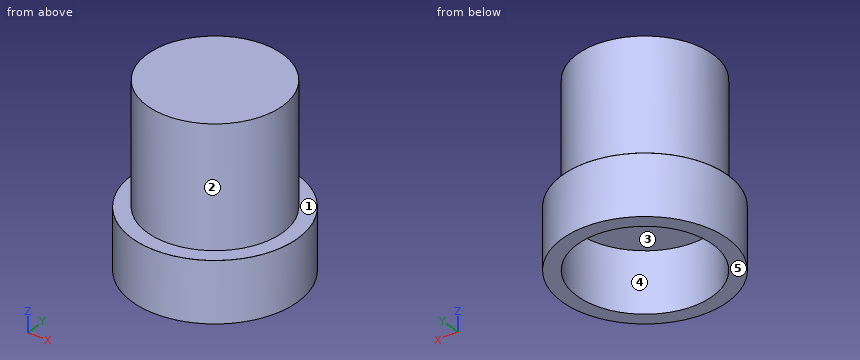
from build123d import *

# Parameters (mm, degrees)
F0_R          = 14.2875
F1_DEPTH      = 25.4
F0_R_2        = 17.4625
F2_DEPTH      = 12.7
F2_DEPTH_BACK = 0.0254


with BuildPart() as f1:
    # F0 (on Top) → F1 (new body)
    with BuildSketch(Plane.XY):
        Circle(F0_R)
    extrude(amount=F1_DEPTH)

    # F0 (on Top) → F2 (join, two sides)
    with BuildSketch(Plane.XY) as f2_sk:
        Circle(F0_R_2)
        Circle(F0_R, mode=Mode.SUBTRACT)
    extrude(amount=-F2_DEPTH)
    extrude(f2_sk.sketch, amount=F2_DEPTH_BACK)


solid = f1.part
Can you work these out from the model? Positions are in its coordinate system, mm. Face numbers are marked on the shaded views. A direction names the side the tool comes from. Coordinates: 2 decimals unless noted, no trailing zeros. Write each loop counter-clockwise with the first axis right and the second up, starting at its lowest first coordinate (ties: lowest second). Pieces come first, ordered by that corner, then holes. Notation, with made-up numbers: M 8,55.25 L 52,55.25 A22 cw 52,71.25 Z; hole C 64,32 d11. An arc over 180 degrees is marked long. Use one line per item in the form item = value.
Q1. We'd pull the mould along Y, two halves only. Please class the marked faces 1, 2 and 3: +Y half, -Y half, draft (parallel to the pull), parting line (faces both ways), or undercut.
Model answer:
face_1 = draft
face_2 = parting line
face_3 = undercut
Q2. If we section it at A-A (x = 0): Write out the boundary of the cut face in (y, z).
Model answer:
outline = M -17.46,-12.7 L -14.29,-12.7 L -14.29,0 L 14.29,0 L 14.29,-12.7 L 17.46,-12.7 L 17.46,0.03 L 14.29,0.03 L 14.29,25.4 L -14.29,25.4 L -14.29,0.03 L -17.46,0.03 Z
Q3. For the marked faces 4 and 5, which set-ups out of +Z, -Z, +X, -X, +Y, -Y let a thin tool reach every point of the face, with its end or its side?
Model answer:
face_4 = -Z
face_5 = -Z, +X, -X, +Y, -Y
Q4. If we section it at D-D (z = 20.5): Write out the boundary of the cut face in (x, y) (1 decimal).
Model answer:
outline = C 0,0 d28.6
Q5. For P1, Ø3, axis at x = 2, z = -2.5, coming from the -Y side; P2, Ø6, axis at y = 14, z = -2, coming from the -X side; P3, Ø6, axis at x = -12.5, z = 15.5, coming from the +Y side, each with a flat end and sliding along its axis, tell me the tip position at first contact or that it passes through.
Model answer:
P1 = -17.46
P2 = -13.56
P3 = 10.67
Q6. I need wall thicknesses on line 1 along Y through (x, z) = (0, -3); line 2 along Y through (x, z) = (-10, -5); line 3 along Z through (x, y) = (-12, -7). Which ranges of each line are inside material? Lowest first, please. Write a range as from..to.
Model answer:
line_1 = -17.46..-14.29, 14.29..17.46
line_2 = -14.32..-10.2, 10.2..14.32
line_3 = 0..25.4
Q7. If we section it at C-C (z = -4): Write out the boundary of the cut face in (x, y) (1 decimal).
Model answer:
outline = C 0,0 d34.9; hole C 0,0 d28.6
